from build123d import *

# Parameters (mm, degrees)
F1_DEPTH  = 850
F3_DEPTH  = 90
F4_W      = 5
F4_H      = 760
F5_DEPTH  = 20
F7_DEPTH  = 20
F8_W      = 570.735931
F8_H      = 5
F9_DEPTH  = 20
F10_W     = 600
F10_H     = 5
F11_DEPTH = 20


with BuildPart() as f1:
    # F0 (on Top) → F1 (new body)
    with BuildSketch(Plane.XY):
        Polygon((-993.667342, 1110.628466), (-993.667342, -939.371534), (-393.667342, -939.371534), (-393.667342, 86.364397), (30.596727, 510.628466), (916.332658, 510.628466), (916.332658, 1110.628466), align=None)
    extrude(amount=F1_DEPTH)

    # F2 (on face) → F3 (cut)
    with BuildSketch(Plane(origin=(0, 0, 0), x_dir=(1, 0, 0), z_dir=(0, 0, -1))):
        Polygon((-993.667342, 919.371534), (-413.667342, 919.371534), (-413.667342, -94.648668), (22.312456, -530.628466), (896.332658, -530.628466), (896.332658, -1110.628466), (916.332658, -1110.628466), (916.332658, -510.628466), (30.596727, -510.628466), (-393.667342, -86.364397), (-393.667342, 939.371534), (-993.667342, 939.371534), align=None)
    extrude(amount=-F3_DEPTH, mode=Mode.SUBTRACT)

    # F4 (on face) → F5 (cut)
    with BuildSketch(Plane.YZ.offset(-393.667342)):
        with Locations((-486.871534, 470)):
            Rectangle(F4_W, F4_H)
    extrude(amount=-F5_DEPTH, mode=Mode.SUBTRACT)

    # F6 (on face) → F7 (cut)
    with BuildSketch(Plane.XZ.offset(-510.628466)):
        Polygon((470.964693, 702.5), (30.596727, 702.5), (30.596727, 697.5), (470.964693, 697.5), (470.964693, 398.75), (30.596727, 398.75), (30.596727, 393.75), (470.964693, 393.75), (470.964693, 90), (475.964693, 90), (475.964693, 393.75), (916.332658, 393.75), (916.332658, 398.75), (475.964693, 398.75), (475.964693, 697.5), (916.332658, 697.5), (916.332658, 702.5), (475.964693, 702.5), (475.964693, 850), (470.964693, 850), align=None)
    extrude(amount=-F7_DEPTH, mode=Mode.SUBTRACT)

    # F8 (on face) → F9 (cut)
    with BuildSketch(Plane.YZ.offset(-393.667342)):
        with Locations((-199.003569, 700)):
            Rectangle(F8_W, F8_H)
        with Locations((-199.003569, 396.25)):
            Rectangle(F8_W, F8_H)
    extrude(amount=-F9_DEPTH, mode=Mode.SUBTRACT)

    # F10 (on face) → F11 (cut)
    with BuildSketch(Plane(origin=(-240.015869, 240.015869, 0), x_dir=(0.707107, 0.707107, 0), z_dir=(0.707107, -0.707107, 0))):
        with Locations((82.704004, 700)):
            Rectangle(F10_W, F10_H)
        with Locations((82.704004, 396.25)):
            Rectangle(F10_W, F10_H)
    extrude(amount=-F11_DEPTH, mode=Mode.SUBTRACT)


solid = f1.part
Model file for the job. Use its own axes, mm. A direction names the side the tool comes from. Round coordinates to 2 decimals unless told otherwise and drop trailing zeros. Order: outer loops, then holes, each group sorted by start corner. A loop starts at its lowest first (then second) coordinate and runs counter-clockwise, first axis right, second up.
(1) Pull direction Z, two halves, no side cores. Call faces 4 (the face through (-198.647, 309.669, 396.285)), 5 (the face through (-272, 335, 0)), 6 (the face through (693, 510.628, 775)), 7 (the face through (-191, 302, 702.5)): released by +Z, released by -Z, zero draft, split by the parting line, or undercut.
(2) Band-saw the part on C-C (x = 675). List the corners of the cut face in (y, z).
(3) Band-saw the part on A-A (y = -263.5). List the corners of the cut face in (x, z).
(4) Band-saw the part on B-B (z = 532). List the corners of the cut face in (x, y).
(5) Pin check, flat tips, straight feed: pin 1 (10 mm diameter, centred on x = 196, y = 518, fed in from -Z); pin 2 (4 mm diameter, centred on x = -527.5, y = 174, fed in from -Z); pin 3 (2.5 mm diameter, centred on y = 522.5, z = 699, fed in from +X); pin 4 (1.5 mm diameter, centred on y = -290, z = 144, fed in from +X). Stop position of each tip, or through.
(6) 3-axis set-ups, long thin cutter, end or side, ignore diameter. For faces 1 (the face through (248, 510.628, 546)), 2 (the face through (-264, 328, 850)), 3 (the face through (-708, -919.372, 44)): which of +Z, -Z, +X, -X, +Y, -Y reach the whole face in a straight line?
(7) Drill centre lines: line 1 (Y direction, x = 100.5, z = 781); line 2 (Y direction, x = 560.5, z = 71.5); line 3 (X direction, y = 39.5, z = 569.5). Where is each one in solid material? Low to high.
(8) Band-saw the part on D-D (y = -597.5). List the corners of the cut face in (x, z), then the cut area to 3 significant figures.
Verdict:
1. face 4: undercut
1. face 5: released by -Z
1. face 6: zero draft
1. face 7: undercut
2. outline: (510.63, 90) - (530.63, 90) - (530.63, 0) - (1110.63, 0) - (1110.63, 850) - (510.63, 850) - (510.63, 702.5) - (530.63, 702.5) - (530.63, 697.5) - (510.63, 697.5) - (510.63, 398.75) - (530.63, 398.75) - (530.63, 393.75) - (510.63, 393.75) - close
3. outline: (-993.67, 0) - (-413.67, 0) - (-413.67, 90) - (-393.67, 90) - (-393.67, 393.75) - (-413.67, 393.75) - (-413.67, 398.75) - (-393.67, 398.75) - (-393.67, 697.5) - (-413.67, 697.5) - (-413.67, 702.5) - (-393.67, 702.5) - (-393.67, 850) - (-993.67, 850) - close
4. outline: (-993.67, -939.37) - (-393.67, -939.37) - (-393.67, -489.37) - (-413.67, -489.37) - (-413.67, -484.37) - (-393.67, -484.37) - (-393.67, 86.36) - (30.6, 510.63) - (470.96, 510.63) - (470.96, 530.63) - (475.96, 530.63) - (475.96, 510.63) - (916.33, 510.63) - (916.33, 1110.63) - (-993.67, 1110.63) - close
5. pin 1: stops at z = 90
5. pin 2: stops at z = 0
5. pin 3: stops at x = 30.6
5. pin 4: stops at x = -393.67
6. face 1: +Z, -Z, +X, -Y
6. face 2: +Z, +X, -X, +Y, -Y
6. face 3: -Z, +X, -X, -Y
7. line 1: y = 510.63 to 1110.63
7. line 2: y = 530.63 to 1110.63
7. line 3: x = -993.67 to -393.67
8. outline: (-993.67, 0) - (-413.67, 0) - (-413.67, 90) - (-393.67, 90) - (-393.67, 850) - (-993.67, 850) - close
8. area: 508,000 mm2
